For this review, take the finished solid that the model builds, in its own axes (mm). Give positions to 0.01 mm unless a question says otherwise; leave off trailing zeros. Write each loop counter-clockwise with the first axis right and the second up, starting at its lowest first coordinate (ties: lowest second). Pieces come first, ordered by that corner, then holes.
from build123d import *

# Parameters (mm, degrees)
SKETCH1_W           = 215.9
SKETCH1_H           = 146.05
SKETCH1_R           = 6.35
SKETCH1_R_2         = 19.05
SKETCH1_R_3         = 3.175
SKETCH1_W_2         = 6.604
SKETCH1_H_2         = 19.05
BOSS_EXTRUDE1_DEPTH = 3.175
SKETCH2_R           = 3.175
CUT_EXTRUDE1_DEPTH  = 7.35
FILLET1_R           = 6.35


with BuildPart() as part:
    # Sketch1 → Boss-Extrude1 (new body, symmetric)
    with BuildSketch(Plane.XY):
        with Locations((-44.45, 0)):
            Rectangle(SKETCH1_W, SKETCH1_H)
        with Locations((50.8, 60.325)):
            Circle(SKETCH1_R, mode=Mode.SUBTRACT)
        with Locations((50.8, -60.325)):
            Circle(SKETCH1_R, mode=Mode.SUBTRACT)
        Circle(SKETCH1_R_2, mode=Mode.SUBTRACT)
        with Locations((0, 45)):
            Circle(SKETCH1_R_3, mode=Mode.SUBTRACT)
        with Locations((0, -45)):
            Circle(SKETCH1_R_3, mode=Mode.SUBTRACT)
        with Locations((-69.85, 60.325)):
            Circle(SKETCH1_R, mode=Mode.SUBTRACT)
        with Locations((-69.85, -60.325)):
            Circle(SKETCH1_R, mode=Mode.SUBTRACT)
        with Locations((-55.88, 0)):
            Rectangle(SKETCH1_W_2, SKETCH1_H_2, mode=Mode.SUBTRACT)
        with Locations((-55.88, 36.5125)):
            Rectangle(SKETCH1_W_2, SKETCH1_H_2, mode=Mode.SUBTRACT)
        with Locations((-55.88, -36.5125)):
            Rectangle(SKETCH1_W_2, SKETCH1_H_2, mode=Mode.SUBTRACT)
    extrude(amount=BOSS_EXTRUDE1_DEPTH, both=True)

    # Sketch2 → Cut-Extrude1 (cut, through all)
    with BuildSketch(Plane.XY.offset(3.175)):
        with Locations((-120.65, -41.275)):
            Circle(SKETCH2_R)
        Polygon((-88.9, 73.025), (-152.4, -15.875), (-152.4, 73.025), align=None)
    extrude(amount=-CUT_EXTRUDE1_DEPTH, mode=Mode.SUBTRACT)

    # Fillet1
    fillet1_edges = [part.edges().sort_by_distance(p)[0] for p in [
        (63.5, 73.025, 0),
        (63.5, -73.025, 0),
        (-152.4, -73.025, 0),
        (-88.9, 73.025, 0),
        (-152.4, -15.875, 0),
    ]]
    fillet(fillet1_edges, radius=FILLET1_R)


solid = part.part
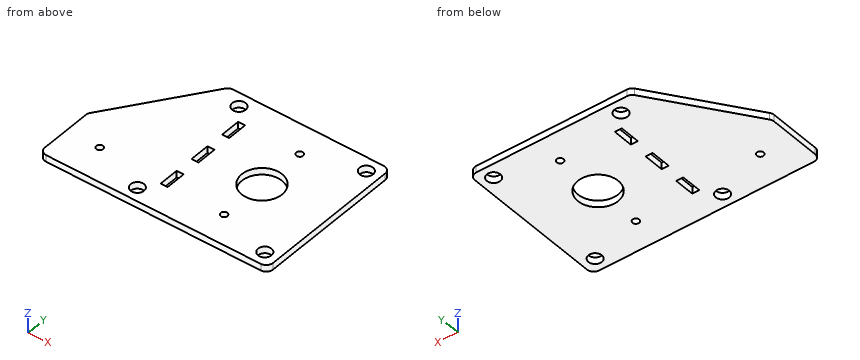
(1) We need section C-C (z = -0.25). Count the separate pieces of the cut face and the enclosed holes in it, and give its area (3 significant figures).
(2) We need section B-B (x = 0). Write out the cut boundary in (y, z) (3 decimals), and give its area (3 significant figures).
(3) For L1, parallel to Y at x = 0, z = -1.5 (3 decimals); L2, parallel to X at y = -61, z = -1.5; L3, parallel to Y at x = -69.85, z = 0.5 (3 decimals), list the stretches that pass through material, from the lowest coordinate up.
(4) We need section A-A (x = 50.8). Write out the cut boundary in (y, z) (3 decimals), and give its area (3 significant figures).
(5) Clearance check with a flat-ended pin moving along its axis: pin 1 Ø3 at (y, z) = (41, -0.5) entering from -X. State where the tip first meets the part, or that it passes through.
(6) We need section D-D (x = -120.65). Write out the cut boundary in (y, z) (3 decimals).
The answers:
1. separate pieces: 1
1. enclosed holes: 11
1. area: 26,600 mm2
2. outline: (-73.025, -3.175) - (-48.175, -3.175) - (-48.175, 3.175) - (-73.025, 3.175) - close; (-41.825, -3.175) - (-19.05, -3.175) - (-19.05, 3.175) - (-41.825, 3.175) - close; (19.05, -3.175) - (41.825, -3.175) - (41.825, 3.175) - (19.05, 3.175) - close; (48.175, -3.175) - (73.025, -3.175) - (73.025, 3.175) - (48.175, 3.175) - close
2. area: 605 mm2
3. L1: y = -73.025 to -48.175, -41.825 to -19.05, 19.05 to 41.825, 48.175 to 73.025
3. L2: x = -152.4 to -76.16, -63.54 to 44.49, 57.11 to 63.5
3. L3: y = -73.025 to -66.675, -53.975 to 53.975, 66.675 to 73.025
4. outline: (-73.025, -3.175) - (-66.675, -3.175) - (-66.675, 3.175) - (-73.025, 3.175) - close; (-53.975, -3.175) - (53.975, -3.175) - (53.975, 3.175) - (-53.975, 3.175) - close; (66.675, -3.175) - (73.025, -3.175) - (73.025, 3.175) - (66.675, 3.175) - close
4. area: 766 mm2
5. pin 1: stops at x = -112.85
6. outline: (-73.025, -3.175) - (-44.45, -3.175) - (-44.45, 3.175) - (-73.025, 3.175) - close; (-38.1, -3.175) - (28.575, -3.175) - (28.575, 3.175) - (-38.1, 3.175) - close
